from build123d import *

# Parameters (mm, degrees)
F0_R     = 5.5
F1_DEPTH = 12
F2_R     = 1.5
F3_DEPTH = 12
F5_DEPTH = 22
F6_R     = 11.5
F7_DEPTH = 3


with BuildPart() as f1:
    # F0 (on Top) → F1 (new body)
    with BuildSketch(Plane.XY):
        Polygon((9.5, 2), (9.5, 13), (-9.5, 13), (-9.5, 2), (-10, 2), (-10, -11), (10, -11), (10, 2), align=None)
        Circle(F0_R, mode=Mode.SUBTRACT)
    extrude(amount=F1_DEPTH)

    # F2 (on face) → F3 (cut)
    with BuildSketch(Plane.XY.offset(12)):
        with Locations((7.75, 0)):
            Circle(F2_R)
        with Locations((-7.75, 0)):
            Circle(F2_R)
        with Locations((0, -8)):
            Circle(F2_R)
    extrude(amount=-F3_DEPTH, mode=Mode.SUBTRACT)

    # F4 (on face) → F5 (cut)
    with BuildSketch(Plane.YZ.offset(9.5)):
        with BuildLine():
            ThreePointArc((9.5, 6), (8, 7.5), (6.5, 6))
            ThreePointArc((6.5, 6), (8, 4.5), (9.5, 6))
        make_face()
    extrude(amount=-F5_DEPTH, mode=Mode.SUBTRACT)

    # F6 (on face) → F7 (cut)
    with BuildSketch(Plane.XY.offset(12)):
        with Locations((0, -1.604815)):
            Circle(F6_R)
    extrude(amount=-F7_DEPTH, mode=Mode.SUBTRACT)


solid = f1.part
Here's how the part is built. I have some questions about the finished solid (model axes, mm). A direction names the side the tool comes from. Round coordinates to 2 decimals unless told otherwise and drop trailing zeros. Loops run counter-clockwise (first coordinate to the right, second up) from the corner with the lowest first, then second, coordinate; pieces in that order, holes last. Notation, with made-up numbers: M -14.75,-11.75 L 43.25,-11.75 A28 cw 43.25,20.25 Z; hole C 0.5,69 d1. An arc over 180 degrees is marked long. Write each question's results on one line, items separated by ' | '. Start each with the question number.
(1) I want a section at C-C (y = 0). Please give me the cut outline in (x, z), then the cut area to 3 significant figures.
(2) On a 3-axis mill with a long thin cutter (end or side, diameter ignored), from which of +Z, -Z, +X, -X, +Y, -Y can I reach the whole of each face in a straight line? I mean faces 1 (the flat face through (9.5, 6, 6)), 2 (the cylindrical face through (0.157, 9.894, 10.521)), 3 (the cylindrical face through (6.25, 0.07, 4.56)). Say none if no direction works.
(3) I want a section at A-A (z = 6). Please give me the cut outline in (x, y).
(4) Thinking about a two-plate mould opening in Y: for faces 4 (the cylindrical face through (-8.545, -9.301, 10.521)), 5 (the flat face through (-9.5, 6, 6)), 6 (the flat face through (0, -11, 5)), 7 (the cylindrical face through (0.13, 9.5, 5.93)), which applies, pulls with the +Y half, pulls with the -Y half, needs draft (parallel to the pull), parting line crosses it, or undercut?
(5) Will these pins go through, and if not, where does the flat tip stop? P1, Ø4, axis at x = 7.75, y = 0, coming from the +Z side; P2, Ø4, axis at y = 8, z = 6, coming from the +X side; P3, Ø3.5, axis at y = 5.5, z = 8.5, coming from the -X side; P4, Ø2.5, axis at x = -7.75, y = 0, coming from the -Z side.
(6) I want a section at B-B (x = 0). Please give me the cut outline in (y, z), then the cut area to 3 significant figures.
(7) If I drill on probe 1 along Y at (x, z) = (8, 6.25); probe 2 along Y at (x, z) = (-8.25, 6); probe 3 along Z at (x, y) = (-3, 6.25), over which ranges is the centre line in solid material (lowest first)? Write a range as from..to.
(8) I want a section at D-D (z = 8). Please give me the cut outline in (x, y), then the cut area to 3 significant figures.
Solved:
1) outline: M -10,0 L -9.25,0 L -9.25,9 L -10,9 Z; M -6.25,0 L -5.5,0 L -5.5,9 L -6.25,9 Z; M 5.5,0 L 6.25,0 L 6.25,9 L 5.5,9 Z; M 9.25,0 L 10,0 L 10,9 L 9.25,9 Z | area: 27.0 mm²
2) face 1: +Z, -Z, +X, +Y | face 2: +Z | face 3: +Z, -Z
3) outline: M -10,-11 L 10,-11 L 10,2 L 9.5,2 L 9.5,6.5 L -9.5,6.5 L -9.5,2 L -10,2 Z; M -9.5,9.5 L 9.5,9.5 L 9.5,13 L -9.5,13 Z; hole C -7.75,0 d3; hole C 0,0 d11; hole C 0,-8 d3; hole C 7.75,0 d3
4) face 4: undercut | face 5: needs draft | face 6: pulls with the -Y half | face 7: undercut
5) P1: stops at z = 9 | P2: stops at x = 9.5 | P3: stops at x = -9.5 | P4: passes through
6) outline: M -11,0 L -9.5,0 L -9.5,9 L -11,9 Z; M -6.5,0 L -5.5,0 L -5.5,9 L -6.5,9 Z; M 5.5,0 L 13,0 L 13,12 L 9.9,12 L 9.9,9 L 5.5,9 Z; hole C 8,6 d3 | area: 92.2 mm²
7) probe 1: y = -11..-1.48, 1.48..6.52, 9.48..13 | probe 2: y = -11..-1.41, 1.41..6.5, 9.5..13 | probe 3: z = 0..9
8) outline: M -10,-11 L 10,-11 L 10,2 L 9.5,2 L 9.5,13 L -9.5,13 L -9.5,2 L -10,2 Z; hole C -7.75,0 d3; hole C 0,0 d11; hole C 0,-8 d3; hole C 7.75,0 d3 | area: 353 mm²
